Work out the finished part from the listing and answer in its coordinate system (mm). Coordinates: 2 decimals unless noted, no trailing zeros. Order: outer loops, then holes, each group sorted by start corner. A loop starts at its lowest first (then second) coordinate and runs counter-clockwise, first axis right, second up. Notation, with made-up numbers: (27, 28) - (68, 28) arc R35 cw to (68, 63) - close; hole circle Ø2 at (20, 17). An arc over 180 degrees is marked (long way). Answer as a JSON object with one key per item and string values. Group by question number.
1) Find the intervals of material crossed by line 1 along X through (y, z) = (-3.75, 8); line 2 along Z through (x, y) = (-4, -4.75); line 3 along X through (y, z) = (5.5, 2), in increasing order.
2) Section C-C (z = 14.25) is taken. Give the vertices of the cut face in (x, y), plus the area to 3 significant figures.
3) The mould has two halves that part along Y. Classify faces 1 (the face through (-8, -8, 8)), 2 (the face through (-8, 8, 8)), 3 (the face through (-16, 0, 8)): released by +Y, released by -Y, zero draft, split by the parting line, or undercut.
4) Each of these flat-tipped pins is pushed along its axis until it touches: P1, Ø6, axis at x = -16.5, y = -3.5, coming from the -Z side; P2, Ø1, axis at x = -0.5, y = -4, coming from the +Z side; P3, Ø3, axis at y = 4.5, z = 7, coming from the +X side. Where does it stop, or does it pass through?
5) Section A-A (x = -21) is taken. Give the vertices of the cut face in (y, z), plus the area to 3 significant figures.
from build123d import *

# Parameters (mm, degrees)
F1_DEPTH = 16
F2_SIZE  = 15.99999


# Not quite as in the source:
# - a fillet or chamfer is up to 0.001 mm smaller than in the source, because OpenCascade refuses the exact size


with BuildPart() as f1:
    # F0 (on Top) → F1 (new body)
    with BuildSketch(Plane.XY):
        Polygon((8, -8), (8, 8), (0, 8), (-8, 8), (-16, 8), (-24, 8), (-24, -8), (-16, -8), (-8, -8), (0, -8), align=None)
    extrude(amount=F1_DEPTH)

    # F2 (size 16 in the source; OpenCascade refuses exactly that, so slightly less here)
    f2_edges = [f1.edges().sort_by_distance(p)[0] for p in [
        (8, 0, 16),
        (-24, 0, 0),
    ]]
    chamfer(f2_edges, length=F2_SIZE)


solid = f1.part
Report:
{
 "1": {"line 1": "x = -16 to 0", "line 2": "z = 0 to 12", "line 3": "x = -10 to 6"},
 "2": {"outline": "(-22.25, -8) - (-6.25, -8) - (-6.25, 8) - (-22.25, 8) - close", "area": "256 mm²"},
 "3": {"face 1": "released by -Y", "face 2": "released by +Y", "face 3": "zero draft"},
 "4": {"P1": "stops at z = 5.5", "P2": "stops at z = 9", "P3": "stops at x = 2.5"},
 "5": {"outline": "(-8, 13) - (8, 13) - (8, 16) - (-8, 16) - close", "area": "48.0 mm²"}
}
